Geometry check sheet. Reference: the model listing, model coordinates, mm. Coordinates: 2 decimals unless noted, no trailing zeros. Write each loop counter-clockwise with the first axis right and the second up, starting at its lowest first coordinate (ties: lowest second). Pieces come first, ordered by that corner, then holes. Notation, with made-up numbers: (66, 39) -> (101, 39) arc R26 ccw to (101, 59) -> close; hole circle Ø1 at (62.25, 84.25). An arc over 180 degrees is marked (long way). Put each result on its own line as item: value. Start each with the question number.
from build123d import *

# Parameters (mm, degrees)
SKETCH1_W           = 400
SKETCH1_H           = 375
BOSS_EXTRUDE1_DEPTH = 1.5
FILLET1_R           = 3
CHAMFER1_SIZE       = 1
SKETCH6_R           = 4.5
CUT_EXTRUDE1_DEPTH  = 10


with BuildPart() as part:
    # Sketch1 → Boss-Extrude1 (new body)
    with BuildSketch(Plane.XY):
        Rectangle(SKETCH1_W, SKETCH1_H)
    extrude(amount=BOSS_EXTRUDE1_DEPTH)

    # Fillet1
    fillet1_edges = [part.edges().sort_by_distance(p)[0] for p in [
        (200, -187.5, 0.75),
        (-200, -187.5, 0.75),
        (-200, 187.5, 0.75),
        (200, 187.5, 0.75),
    ]]
    fillet(fillet1_edges, radius=FILLET1_R)

    # Chamfer1
    chamfer1_edges = [part.edges().sort_by_distance(p)[0] for p in [
        (0, -187.5, 1.5),
        (-200, 0, 1.5),
        (200, 0, 1.5),
        (0, 187.5, 1.5),
        (-199.121320344, 186.621320344, 1.5),
        (199.121320344, 186.621320344, 1.5),
        (199.121320344, -186.621320344, 1.5),
        (-199.121320344, -186.621320344, 1.5),
    ]]
    chamfer(chamfer1_edges, length=CHAMFER1_SIZE)

    # Sketch6 → Cut-Extrude1 (cut)
    with BuildSketch(Plane.XY.offset(1.5)):
        with Locations((-30, 120)):
            Circle(SKETCH6_R)
        with Locations((30, 120)):
            Circle(SKETCH6_R)
        with Locations((162.8, 30)):
            Circle(SKETCH6_R)
        with Locations((162.8, -30)):
            Circle(SKETCH6_R)
        with Locations((30, -120)):
            Circle(SKETCH6_R)
        with Locations((-30, -120)):
            Circle(SKETCH6_R)
        with Locations((-162.8, 30)):
            Circle(SKETCH6_R)
        with Locations((-162.8, -30)):
            Circle(SKETCH6_R)
    extrude(amount=-CUT_EXTRUDE1_DEPTH, mode=Mode.SUBTRACT)


solid = part.part
Item 1: Go/stop test with a flat-tipped pin: P1, Ø5.5, axis at x = 162.8, y = -30, coming from the +Z side. Record where the tip stops, or that it passes through.
Item 2: Scan lines: line 1 along Y through (x, z) = (-162.8, 0.4); line 2 along Y through (x, z) = (162.8, 1.05); line 3 along Y through (x, z) = (-48, 0.55). Record each from-to range of solid material in increasing order. Write a range as [from, to].
Item 3: Mould release check, pull along Y, two halves, no side actions. Record for faces 1 (the cylindrical face through (32.08, -123.99, 0.76)), 2 (the flat face through (-3, 3, 0)): released by +Y, released by -Y, zero draft, split by the parting line, or undercut.
Item 4: Section check B-B, the plane x = 30. Enter the section's corners in (y, z).
Item 5: Section check A-A, the plane y = -30. Enter the section's corners in (x, z), and give its area (3 significant figures).
From the geometry:
1. P1: through
2. line 1: [-187.5, -34.5], [-25.5, 25.5], [34.5, 187.5]
2. line 2: [-186.95, -34.5], [-25.5, 25.5], [34.5, 186.95]
2. line 3: [-187.45, 187.45]
3. face 1: undercut
3. face 2: zero draft
4. outline: (-187.5, 0) -> (-124.5, 0) -> (-124.5, 1.5) -> (-186.5, 1.5) -> (-187.5, 0.5) -> close; (-115.5, 0) -> (115.5, 0) -> (115.5, 1.5) -> (-115.5, 1.5) -> close; (124.5, 0) -> (187.5, 0) -> (187.5, 0.5) -> (186.5, 1.5) -> (124.5, 1.5) -> close
5. outline: (-200, 0) -> (-167.3, 0) -> (-167.3, 1.5) -> (-199, 1.5) -> (-200, 0.5) -> close; (-158.3, 0) -> (158.3, 0) -> (158.3, 1.5) -> (-158.3, 1.5) -> close; (167.3, 0) -> (200, 0) -> (200, 0.5) -> (199, 1.5) -> (167.3, 1.5) -> close
5. area: 572 mm²
